Here's how the part is built. I have some questions about the finished solid (model axes, mm). Face numbers are marked on the shaded views. A direction names the side the tool comes from. Give positions to 0.01 mm unless a question says otherwise; leave off trailing zeros. Write each loop counter-clockwise with the first axis right and the second up, starting at its lowest first coordinate (ties: lowest second). Pieces come first, ordered by that corner, then holes. Notation, with made-up numbers: (-3.5, 72.5) - (16.5, 72.5) arc R7 cw to (16.5, 76.5) - close; hole circle Ø4 at (-22.5, -11). An arc over 180 degrees is marked (long way). Use a Markdown table: item, result.
```python
from build123d import *

# Parameters (mm, degrees)
F1_DEPTH = 6
F2_T     = -0.25
F3_W     = 1.8021183787
F3_H     = 0.7201734115
F4_DEPTH = 5
F5_W     = 1.6065204982
F5_H     = 0.6512082182
F6_DEPTH = 0.762


with BuildPart() as f1:
    # F0 (on Front) → F1 (new body)
    with BuildSketch(Plane.XZ):
        Polygon((4, -0.5), (4, 1.5), (-4, 1.5), (-4, -0.5), (-3, -1.5), (3, -1.5), align=None)
    extrude(amount=F1_DEPTH)

    # F2
    f2_openings = [f1.faces().sort_by_distance(p)[0] for p in [
        (0, -6, 0.050725),
    ]]
    offset(amount=F2_T, openings=f2_openings)

    # F3 (on face) → F4 (join)
    with BuildSketch(Plane.XZ.offset(0.25)):
        with Locations((-0.9010591893, 0.3600867058)):
            Rectangle(F3_W, F3_H)
        with Locations((0.9010591893, 0.3600867058)):
            Rectangle(F3_W, F3_H)
    extrude(amount=F4_DEPTH)

    # F5 (on face) → F6 (join)
    with BuildSketch(Plane(origin=(0, 0, 0), x_dir=(-1, 0, 0), z_dir=(0, 1, 0))):
        with Locations((0.8032602491, 0.3256041091)):
            Rectangle(F5_W, F5_H)
        with Locations((-0.8032602491, 0.3256041091)):
            Rectangle(F5_W, F5_H)
    extrude(amount=F6_DEPTH)


solid = f1.part
```
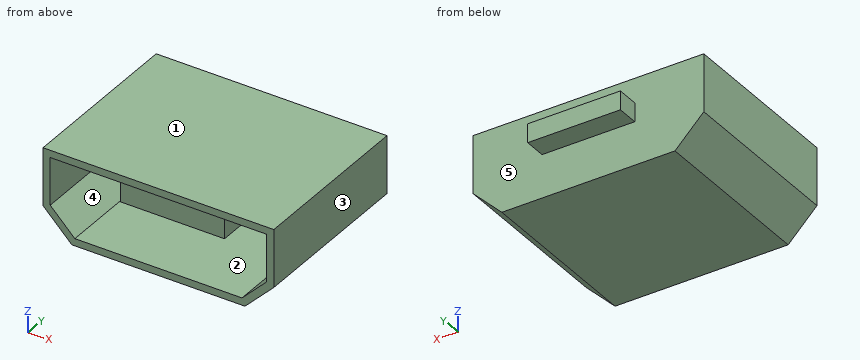
Item 1: For the marked faces 1 and 2, which set-ups out of +Z, -Z, +X, -X, +Y, -Y let a thin tool reach every point of the face, with its end or its side?
Values:
| item | result |
|---|---|
| face 1 | +Z, +X, -X, +Y, -Y |
| face 2 | -Y |
Item 2: Thinking about a two-plate mould opening in X: for the marked faces 3, 4 and 5, which applies, +X half, -X half, draft (parallel to the pull), parting line (faces both ways), or undercut?
Values:
| item | result |
|---|---|
| face 3 | +X half |
| face 4 | undercut |
| face 5 | draft |
Item 3: If we section it at D-D, the plane x = -1.5: Write out the boundary of the cut face in (y, z), plus the area to 3 significant figures.
Values:
| item | result |
|---|---|
| outline | (-6, -1.5) - (0, -1.5) - (0, 0) - (0.76, 0) - (0.76, 0.65) - (0, 0.65) - (0, 1.5) - (-6, 1.5) - (-6, 1.25) - (-0.25, 1.25) - (-0.25, 0.72) - (-5.25, 0.72) - (-5.25, 0) - (-0.25, 0) - (-0.25, -1.25) - (-6, -1.25) - close |
| area | 7.72 mm2 |
Item 4: If we section it at A-A, the plane y = -2: Write out the boundary of the cut face in (x, z), plus the area to 3 significant figures.
Values:
| item | result |
|---|---|
| outline | (-4, -0.5) - (-3, -1.5) - (3, -1.5) - (4, -0.5) - (4, 1.5) - (-4, 1.5) - close; (-1.8, 0) - (1.8, 0) - (1.8, 0.72) - (-1.8, 0.72) - close; hole (-3.75, -0.4) - (-2.9, -1.25) - (2.9, -1.25) - (3.75, -0.4) - (3.75, 1.25) - (-3.75, 1.25) - close |
| area | 7.57 mm2 |
Item 5: I need wall thicknesses on line 1 along Z through (x, y) = (-1.75, -1.75); line 2 along X through (y, z) = (-3, 0.6); line 3 along X through (y, z) = (-2.75, -0.25). Which ranges of each line are inside material? Lowest first, please. Write a range as [from, to].
Values:
| item | result |
|---|---|
| line 1 | z = [-1.5, -1.25], [0, 0.72], [1.25, 1.5] |
| line 2 | x = [-4, -3.75], [-1.8, 1.8], [3.75, 4] |
| line 3 | x = [-4, -3.75], [3.75, 4] |
Item 6: Will these pins go through, and if not, where does the flat tip stop? pin 1 Ø0.6 at (x, y) = (0, 0.5) entering from -Z; pin 2 Ø1.2 at (x, z) = (-0.5, 0) entering from -Y; pin 3 Ø0.5 at (y, z) = (0.5, 0.5) entering from +X; pin 4 Ø1.5 at (y, z) = (0, -1) entering from -X.
Values:
| item | result |
|---|---|
| pin 1 | stops at z = 0 |
| pin 2 | stops at y = -5.25 |
| pin 3 | stops at x = 1.61 |
| pin 4 | stops at x = -4 |
Item 7: If we section it at C-C, the plane x = 2.5: Write out the boundary of the cut face in (y, z).
Values:
| item | result |
|---|---|
| outline | (-6, -1.5) - (0, -1.5) - (0, 1.5) - (-6, 1.5) - (-6, 1.25) - (-0.25, 1.25) - (-0.25, -1.25) - (-6, -1.25) - close |
Item 8: If we section it at B-B, the plane z = 1.15: Write out the boundary of the cut face in (x, y), plus the area to 4 significant figures.
Values:
| item | result |
|---|---|
| outline | (-4, -6) - (-3.75, -6) - (-3.75, -0.25) - (3.75, -0.25) - (3.75, -6) - (4, -6) - (4, 0) - (-4, 0) - close |
| area | 4.875 mm2 |
